Autodesk Inventor part; units mm, degrees
ref_plane "YZ Plane" through (0, 0, 0) normal (1, 0, 0) x (0, 1, 0)
ref_plane "XZ Plane" through (0, 0, 0) normal (0, 1, 0) x (-1, 0, 0)
ref_plane "XY Plane" through (0, 0, 0) normal (0, 0, 1) x (1, 0, 0)
sketch "Эскиз1" plane through (0, 0, 0) normal (0, 1, 0) x (-1, 0, 0)
  line L0 (7.5, 22) -> (-7.5, 22)
  line L1 (-7.5, 22) -> (-7.5, -22)
  line L2 (-7.5, -22) -> (7.5, -22)
  line L3 (7.5, -22) -> (7.5, 22)
  line L4 (-7.5, 22) -> (7.5, -22) construction
  line L5 (0, 22) -> (0, -22) construction
  circle A0 centre (0, 16) radius 2
  line L6 (7.5, 0) -> (-7.5, 0) construction
  circle A1 centre (0, -16) radius 2
  point P0 (0, 0)
  point P1 (0, 0)
  dimension "d0" = 15
  dimension "d1" = 44
  dimension "d2" = 16
  dimension "d3" = 4
extrude "Выдавливание1" add sketch "Эскиз1" along normal blind 14.7
sketch "Эскиз2" plane through (7.5, 0, 22) normal (1, 0, 0) x (0, 0, -1)
  line L0 (0, 14.7) -> (44, 14.7)
  circle A0 centre (22, 14.7) radius 10.15
  point P0 (22, 0)
  dimension "Диаметр_мотора" = 20.3
extrude "Выдавливание2" cut sketch "Эскиз2" against normal through all
properties part number "motor_mount_edge_part2-01"
Check sheet for the modelled part. Datum: model origin and axes. Units: mm. Coordinates: 2 decimals unless noted, no trailing zeros. Write each loop counter-clockwise with the first axis right and the second up, starting at its lowest first coordinate (ties: lowest second). Pieces come first, ordered by that corner, then holes. Notation, with made-up numbers: M 35.25,79.5 L 58.25,79.5 A25 ccw 58.25,93.5 Z; hole C 18.25,1 d8. An arc over 180 degrees is marked long. Use one line per item in the form item = value.
Item 1: Sectioned sample at B-B, the plane x = 0. Record the cut outline in (y, z), and give its area (3 significant figures).
Answer below:
outline = M 0,-22 L 14.7,-22 L 14.7,-18 L 0,-18 Z; M 0,-14 L 14.7,-14 L 14.7,-10.15 A10.15 cw 14.7,10.15 L 14.7,14 L 0,14 Z; M 0,18 L 14.7,18 L 14.7,22 L 0,22 Z
area = 367 mm^2
Item 2: Sectioned sample at C-C, the plane y = 10.5. Record the cut outline in (x, z), and give its area (3 significant figures).
Answer below:
outline = M -7.5,-22 L 7.5,-22 L 7.5,-9.24 L -7.5,-9.24 Z; M -7.5,9.24 L 7.5,9.24 L 7.5,22 L -7.5,22 Z; hole C 0,-16 d4; hole C 0,16 d4
area = 358 mm^2
Item 3: Sectioned sample at A-A, the plane z = 16. Record the cut outline in (x, y).
Answer below:
outline = M -7.5,0 L -2,0 L -2,14.7 L -7.5,14.7 Z; M 2,0 L 7.5,0 L 7.5,14.7 L 2,14.7 Z
Item 4: Sectioned sample at D-D, the plane y = 2. Record the cut outline in (x, z), and give its area (3 significant figures).
Answer below:
outline = M -7.5,-22 L 7.5,-22 L 7.5,22 L -7.5,22 Z; hole C 0,-16 d4; hole C 0,16 d4
area = 635 mm^2
Item 5: Release check for a two-part mould opening along Z. For faces 1 (the face through (7.5, 4, 0)), 2 (the face through (0.105, 4.552, 0.223)), 3 (the face through (0, 7, 14)), 4 (the face through (0, 7, -22)) record: pulls with the +Z half, pulls with the -Z half, needs draft (parallel to the pull), parting line crosses it, or undercut.
Answer below:
face_1 = needs draft
face_2 = undercut
face_3 = undercut
face_4 = pulls with the -Z half
Item 6: Material ranges on L1, parallel to Z at x = 0, y = 3.5; L2, parallel to Z at x = 0, y = 6.5; L3, parallel to Z at x = 0, y = 6.25, recorded low to high. Write a range as from..to.
Answer below:
L1 = -22..-18, -14..14, 18..22
L2 = -22..-18, -14..-5.98, 5.98..14, 18..22
L3 = -22..-18, -14..-5.62, 5.62..14, 18..22
